```python
from build123d import *

# Parameters (mm, degrees)
F0_R     = 20.955
F1_DEPTH = 182.88
F2_R     = 12.1285
F3_DEPTH = 37.338
F4_R     = 7.62
F5_R     = 12.1666
F6_DEPTH = 38.1
F7_R     = 7.62


with BuildPart() as f1:
    # F0 (on Top) → F1 (new body)
    with BuildSketch(Plane.XY):
        Circle(F0_R)
    extrude(amount=F1_DEPTH)

    # F2 (on face) → F3 (join)
    with BuildSketch(Plane(origin=(0, 0, 0), x_dir=(1, 0, 0), z_dir=(0, 0, -1))):
        Circle(F2_R)
    extrude(amount=F3_DEPTH)

    # F4
    f4_edges = [f1.edges().sort_by_distance(p)[0] for p in [
        (-12.1285, 0, -37.338),
    ]]
    fillet(f4_edges, radius=F4_R)

    # F5 (on face) → F6 (cut)
    with BuildSketch(Plane.XY.offset(182.88)):
        Circle(F5_R)
    extrude(amount=-F6_DEPTH, mode=Mode.SUBTRACT)

    # F7
    f7_edges = [f1.edges().sort_by_distance(p)[0] for p in [
        (-12.1666, 0, 144.78),
    ]]
    fillet(f7_edges, radius=F7_R)


solid = f1.part
```
Verification items for the finished model (mm, model axes). A direction names the side the tool comes from. Coordinates: 2 decimals unless noted, no trailing zeros. Loops run counter-clockwise (first coordinate to the right, second up) from the corner with the lowest first, then second, coordinate; pieces in that order, holes last. Notation, with made-up numbers: (-34, 44.5) - (18, 44.5) arc R21 ccw to (18, 73.5) - close; hole circle Ø9 at (-5, -1.5). An arc over 180 degrees is marked (long way). Return JSON: item names as keys, results as strings.
1. Section check C-C, the plane z = -14.5. Record the boundary of the cut face in (x, y).
Established:
{"outline": "circle Ø24.26 at (0, 0)"}
2. Tool access check on faces 5 (the flat face through (9, -9, 182.88)), 6 (the flat face through (9, -9, 0)). Record the directions out of +Z, -Z, +X, -X, +Y, -Y that give a thin tool (end or side, any length) a straight path to the whole face; none if there is none.
Established:
{"face 5": "+Z, +X, -X, +Y, -Y", "face 6": "-Z"}
3. Mould release check, pull along X, two halves, no side actions. Record for faces 1 (the flat face through (0, 0, 144.78)), 2 (the cylindrical face through (-2, 12, 168)), 3 (the flat face through (0, 0, -37.338)), 4 (the cylindrical face through (-2.728, 20.777, 90.16)): +X half, -X half, draft (parallel to the pull), parting line (faces both ways), or undercut.
Established:
{"face 1": "undercut", "face 2": "undercut", "face 3": "draft", "face 4": "parting line"}
4. Section check A-A, the plane z = 25.5. Record the boundary of the cut face in (x, y) (3 decimals), then the cut area to 3 significant figures.
Established:
{"outline": "circle Ø41.91 at (0, 0)", "area": "1,380 mm2"}
5. Section check B-B, the plane x = 17.5. Record the boundary of the cut face in (y, z).
Established:
{"outline": "(-11.53, 0) - (11.53, 0) - (11.53, 182.88) - (-11.53, 182.88) - close"}
6. Section check D-D, the plane y = -15.5. Record the boundary of the cut face in (x, z), then the cut area to 3 significant figures.
Established:
{"outline": "(-14.1, 0) - (14.1, 0) - (14.1, 182.88) - (-14.1, 182.88) - close", "area": "5,160 mm2"}
7. Go/stop test with flat-tipped pins: pin 1 (10 mm diameter, centred on x = -9, z = 123.5, fed in from +Y); pin 2 (5 mm diameter, centred on y = 11.5, z = 75, fed in from -X); pin 3 (6 mm diameter, centred on y = 11, z = 100, fed in from +X). Record where each tip stops, or that it passes through.
Established:
{"pin 1": "stops at y = 20.57", "pin 2": "stops at x = -18.92", "pin 3": "stops at x = 19.37"}
8. Thickness scan on L1, parallel to Y at x = 0, z = 172.5 (3 decimals); L2, parallel to Z at x = 3.5, y = 19.5; L3, parallel to Y at x = 17.5, z = 86. Record the ranges inside material, lowest first.
Established:
{"L1": "y = -20.955 to -12.167, 12.167 to 20.955", "L2": "z = 0 to 182.88", "L3": "y = -11.53 to 11.53"}
